The listing builds one solid part. Answer for the finished solid, in the listing's coordinates (mm). A direction names the side the tool comes from. Coordinates: 2 decimals unless noted, no trailing zeros. Order: outer loops, then holes, each group sorted by start corner. A loop starts at its lowest first (then second) coordinate and runs counter-clockwise, first axis right, second up. Notation, with made-up numbers: (-23.75, 12.5) -> (20.25, 12.5) arc R32 cw to (20.25, 47.5) -> close; hole circle Ø9 at (88, 16.5). An arc over 180 degrees is marked (long way). Put each result on its own line as item: value. Start each with the question number.
```python
from build123d import *

# Parameters (mm, degrees)
SKETCH1_R               = 1.9
BOSS_EXTRUDE1_DEPTH     = 1.75
SKETCH2_R               = 1.5
BOSS_EXTRUDE2_DEPTH     = 9
BOSS_EXTRUDE3_START     = 9
SKETCH4_R               = 1.5
BOSS_EXTRUDE3_DEPTH     = 9
CUT_EXTRUDE1_DEPTH      = 12.08072651
CUT_EXTRUDE1_DEPTH_BACK = 12.08072651
CUT_EXTRUDE2_DEPTH      = 6.25
CUT_EXTRUDE3_START      = -3
CUT_EXTRUDE3_DEPTH      = 3


with BuildPart() as part:
    # Sketch1 → Boss-Extrude1 (new, symmetric)
    with BuildSketch(Plane(origin=(0, 0, 0), x_dir=(1, 0, 0), z_dir=(0, 1, 0))):
        with Locations(Location((0, 0, 0), (0, 0, 270))):
            Circle(SKETCH1_R)
    extrude(amount=BOSS_EXTRUDE1_DEPTH, both=True)

    # Sketch2 → Boss-Extrude2 (add)
    with BuildSketch(Plane.XZ.offset(1.75)):
        with Locations(Location((0, 0, 0), (0, 0, 270))):
            Circle(SKETCH2_R)
    extrude(amount=BOSS_EXTRUDE2_DEPTH)

    # Sketch4 → Boss-Extrude3 (add)
    with BuildSketch(Plane(origin=(0, 1.75, 0), x_dir=(1, 0, 0), z_dir=(0, 1, 0)).offset(BOSS_EXTRUDE3_START)):
        with Locations(Location((0, 0, 0), (0, 0, 90))):
            Circle(SKETCH4_R)
    extrude(amount=-BOSS_EXTRUDE3_DEPTH)

    # Sketch3 → Cut-Extrude1 (cut, two sides: drawn at the far end of the back side and taken through both)
    with BuildSketch(Plane(origin=(0, 0, 0), x_dir=(1, 0, 0), z_dir=(0, 1, 0)).offset(-CUT_EXTRUDE1_DEPTH_BACK)):
        with BuildLine():
            Line((-1.549193338, 1.1), (1.549193338, 1.1))
            ThreePointArc((1.549193338, 1.1), (0, 1.9), (-1.549193338, 1.1))
        make_face()
    extrude(amount=CUT_EXTRUDE1_DEPTH + CUT_EXTRUDE1_DEPTH_BACK, mode=Mode.SUBTRACT)

    # Sketch5 → Cut-Extrude2 (cut)
    with BuildSketch(Plane(origin=(0, 10.75, 0), x_dir=(1, 0, 0), z_dir=(0, 1, 0))):
        with BuildLine():
            Line((1.019803903, -1.1), (-1.019803903, -1.1))
            ThreePointArc((-1.019803903, -1.1), (0, -1.5), (1.019803903, -1.1))
        make_face()
    extrude(amount=-CUT_EXTRUDE2_DEPTH, mode=Mode.SUBTRACT)

    # Sketch6 → Cut-Extrude3 (cut)
    with BuildSketch(Plane.XZ.offset(10.75).offset(CUT_EXTRUDE3_START)):
        with BuildLine():
            Line((-1.019803903, 1.1), (1.019803903, 1.1))
            ThreePointArc((1.019803903, 1.1), (0, 1.5), (-1.019803903, 1.1))
        make_face()
    extrude(amount=CUT_EXTRUDE3_DEPTH, mode=Mode.SUBTRACT)


solid = part.part
```
(1) The part is cut by section A-A on x = 0. Determine the outline of the cut face in (y, z), plus the area to 3 significant figures.
(2) Find the intervals of material crossed by L1, parallel to Z at x = -0.4, y = 4.75; L2, parallel to X at y = 7.5, z = 0; L3, parallel to Y at x = 0.45, z = 1.5, in increasing order.
(3) The part is cut by section B-B on z = 0. Determine the outline of the cut face in (x, y).
(4) The part is cut by section C-C on y = 6.5. Determine the outline of the cut face in (x, z), plus the area to 3 significant figures.
(5) A tool of negligible diameter and unlimited length cuts with its end or side. For faces 1 (the flat face through (0, -9, 1.1)), 2 (the flat face through (0, 8, 1.1)), 3 (the cylindrical face through (0.05, -6.19, 1.5)), 4 (the cylindrical face through (1.286, 6.313, 0.772)), from which of +Z, -Z, +X, -X, +Y, -Y can it reach the whole face along a straight path? Write none if from no direction.
(6) Each of these flat-tipped pins is pushed along its axis until it touches: P1, Ø2, axis at x = 0.5, y = -9.5, coming from the +Z side; P2, Ø1.5, axis at x = 0, z = 1.5, coming from the -Y side. Where does it stop, or does it pass through?
Worked out:
1. outline: (-10.75, -1.1) -> (10.75, -1.1) -> (10.75, 1.1) -> (4.5, 1.1) -> (4.5, 1.5) -> (1.75, 1.5) -> (1.75, 1.9) -> (-1.75, 1.9) -> (-1.75, 1.5) -> (-7.75, 1.5) -> (-7.75, 1.1) -> (-10.75, 1.1) -> close
1. area: 53.6 mm2
2. L1: -1.1 to 1.1
2. L2: -1.5 to 1.5
2. L3: -1.75 to 1.75
3. outline: (-1.9, -1.75) -> (-1.5, -1.75) -> (-1.5, -10.75) -> (1.5, -10.75) -> (1.5, -1.75) -> (1.9, -1.75) -> (1.9, 1.75) -> (1.5, 1.75) -> (1.5, 10.75) -> (-1.5, 10.75) -> (-1.5, 1.75) -> (-1.9, 1.75) -> close
4. outline: (-1.02, -1.1) -> (1.02, -1.1) arc R1.5 ccw to (1.02, 1.1) -> (-1.02, 1.1) arc R1.5 ccw to start
4. area: 5.95 mm2
5. face 1: +Z, +X, -X, -Y
5. face 2: +Z, +X, -X, +Y
5. face 3: -Y
5. face 4: +Y
6. P1: z = 1.1
6. P2: y = -10.75
